For this review, use the dimensioned drawing (mm, ordinates from the lowest corner) and the shaded views. Coordinates: 2 decimals unless noted, no trailing zeros. Loops run counter-clockwise (first coordinate to the right, second up) from the corner with the lowest first, then second, coordinate; pieces in that order, holes last. Notation, with made-up numbers: M 54.5,40.5 L 92.5,40.5 A17 ccw 92.5,51.5 Z; hole C 66.5,-24 d6. An arc over 180 degrees is marked long. One line per item, written item: value.
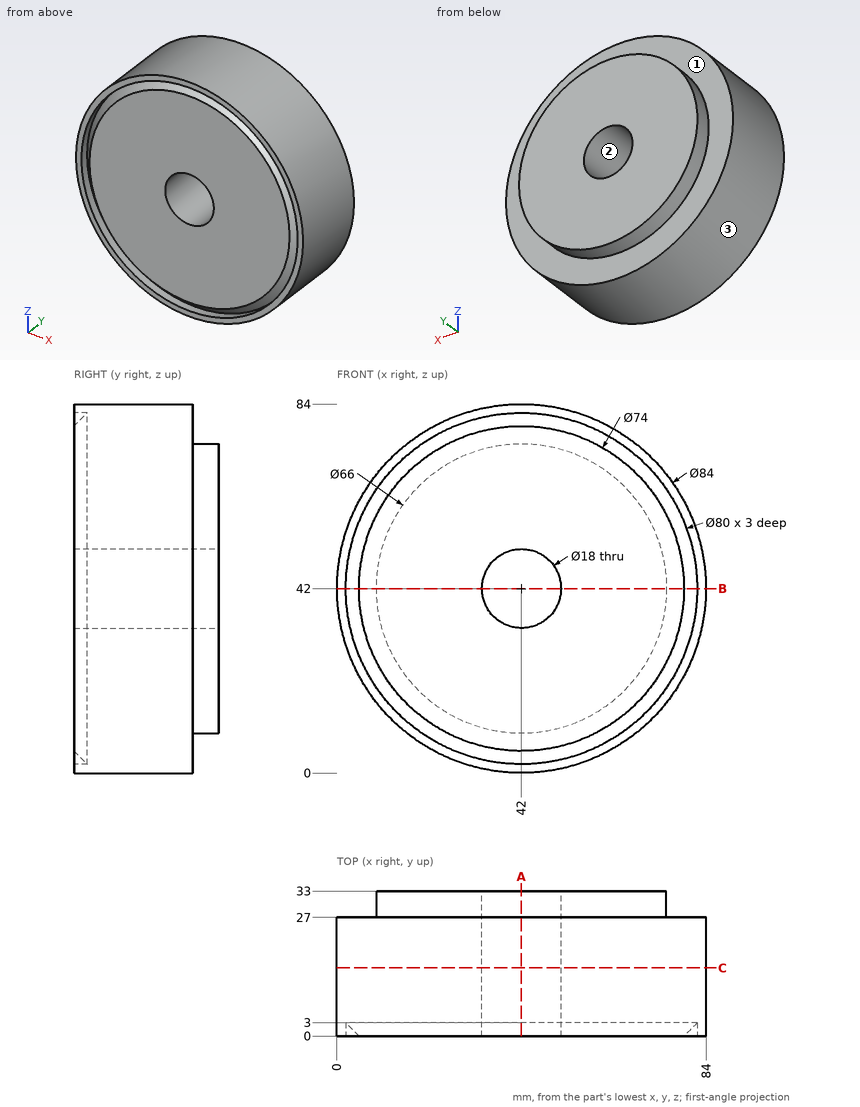
(1) Insertion check: pin 1 (2 mm diameter, centred on y = 26, z = 22.5, fed in from -X); pin 2 (3 mm diameter, centred on x = 34, y = 10, fed in from -Z); pin 3 (12 mm diameter, centred on y = 28, z = 16.5, fed in from +X). Each pin has a flat end and moves straight along its axis. Give the tip position at first contact, or say it passes through.
Reply:
pin 1: stops at x = 4.29
pin 2: stops at z = 0.51
pin 3: stops at x = 79.15
(2) We need section C-C on y = 15.5. State the section outline as (x, z) points.
Reply:
outline: C 42,42 d84; hole C 42,42 d18
(3) We need section A-A on x = 42. State the section outline as (y, z) points, then the cut area to 3 significant figures.
Reply:
outline: M 0,0 L 27,0 L 27,9 L 33,9 L 33,33 L 0,33 L 0,5 L 3,2 L 0,2 Z; M 0,51 L 33,51 L 33,75 L 27,75 L 27,84 L 0,84 L 0,82 L 3,82 L 0,79 Z
area: 2,060 mm2
(4) Mouldability with a two-part tool opening along Z and no side actions: class the marked faces 1, 2 and 3 as released by +Z, released by -Z, zero draft, split by the parting line, or undercut.
Reply:
face 1: zero draft
face 2: undercut
face 3: split by the parting line
(5) We need section B-B on z = 42. State the section outline as (x, y) points, then the cut area to 3 significant figures.
Reply:
outline: M 0,0 L 2,0 L 2,3 L 5,0 L 33,0 L 33,33 L 9,33 L 9,27 L 0,27 Z; M 51,0 L 79,0 L 82,3 L 82,0 L 84,0 L 84,27 L 75,27 L 75,33 L 51,33 Z
area: 2,060 mm2
(6) To check wall thickness, follow line 1 along Z through (x, y) = (42, 0.7); line 2 along X through (y, z) = (1.3, 42); line 3 along X through (y, z) = (2.45, 42). State the ranges of each line that lie inside material, in increasing order. Write a range as [from, to].
Reply:
line 1: z = [0, 2], [4.3, 33], [51, 79.7], [82, 84]
line 2: x = [0, 2], [3.7, 33], [51, 80.3], [82, 84]
line 3: x = [0, 2], [2.55, 33], [51, 81.45], [82, 84]
